```python
from build123d import *

# Parameters (mm, degrees)
BOSS_EXTRUDE1_DEPTH        = 32.1564
SKETCH2_W                  = 57.9628
SKETCH2_H                  = 20.955
CUT_EXTRUDE1_DEPTH         = 80.772
F_31_0_12_DIAMETER_HOLE1_D = 3.048
F_2_0_221_DIAMETER_HOLE1_D = 5.6134
FILLET1_R                  = 2.54


with BuildPart() as part:
    # Sketch1 → Boss-Extrude1 (new body, symmetric)
    with BuildSketch(Plane(origin=(0, 0, 0), x_dir=(0, 0, -1), z_dir=(1, 0, 0))):
        Polygon((0, 0), (24.13, 0), (9.4742, 83.947), (0, 83.947), align=None)
    extrude(amount=BOSS_EXTRUDE1_DEPTH, both=True)

    # Sketch2 → Cut-Extrude1 (cut)
    with BuildSketch(Plane(origin=(0, 83.947, 0), x_dir=(1, 0, 0), z_dir=(0, 1, 0))):
        with Locations((0, 13.6525)):
            Rectangle(SKETCH2_W, SKETCH2_H)
    extrude(amount=-CUT_EXTRUDE1_DEPTH, mode=Mode.SUBTRACT)

    # #31 (0.12) Diameter Hole1 (through all)
    with Locations(Plane.XY):
        with Locations((-21.971, 74.3331), (22.0472, 74.3331), (22.0472, 10.668), (-21.971, 10.668)):
            Hole(F_31_0_12_DIAMETER_HOLE1_D / 2)

    # #2 (0.221) Diameter Hole1 (through all)
    with Locations(Plane(origin=(0, 0, 0), x_dir=(-1, 0, 0), z_dir=(0, -1, 0))):
        with Locations((-16.9164, 12.065), (16.9164, 12.065)):
            Hole(F_2_0_221_DIAMETER_HOLE1_D / 2)

    # Fillet1
    fillet1_edges = [part.edges().sort_by_distance(p)[0] for p in [
        (0, 3.175, -23.575695915),
        (28.9814, 43.561, -16.524947958),
        (-28.9814, 43.561, -16.524947958),
        (-28.9814, 43.561, -3.175),
        (-28.9814, 83.947, -6.3246),
        (0, 83.947, -3.175),
        (28.9814, 83.947, -6.3246),
        (28.9814, 3.175, -13.375347958),
        (0, 3.175, -3.175),
        (-28.9814, 3.175, -13.375347958),
        (28.9814, 43.561, -3.175),
    ]]
    fillet(fillet1_edges, radius=FILLET1_R)


solid = part.part
```
Design review of the part built by this model. Coordinates are the model's own, in mm. A direction names the side the tool comes from. Coordinates: 2 decimals unless noted, no trailing zeros. Order: outer loops, then holes, each group sorted by start corner. A loop starts at its lowest first (then second) coordinate and runs counter-clockwise, first axis right, second up.
1) Mouldability with a two-part tool opening along X and no side actions: class faces 3 (the flat face through (0.2, 83.947, -0.2)), 4 (the flat face through (-32.156, 33, -9)), 5 (the flat face through (-28.981, 36, -11)) as +X half, -X half, draft (parallel to the pull), parting line (faces both ways), or undercut.
2) Take a section at B-B, the plane x = -16. Give the boundary of the cut face in (y, z) (3 decimals).
3) Clearance check with flat-ended pins moving along their axes: pin 1 (12 mm diameter, centred on x = 5.5, z = -19, fed in from +Y) (3 decimals); pin 2 (5 mm diameter, centred on x = 22.05, y = 10.67, fed in from -Z) (3 decimals). State where each tip first meets the part, or that it passes through.
4) For faces 1 (the cylindrical face through (-20.848, 75.363, -1.61)), 2 (the cylindrical face through (29.7, 44.4, -15.6)), list the 3-axis set-ups (+Z, -Z, +X, -X, +Y, -Y) from which the entire face can be reached by the end or side of a thin tool; tool diameter is ignored.
5) Take a section at C-C, the plane z = -13.5. State how many separate pieces and enclosed holes the cut face has, and give its area (3 significant figures).
6) Wall thickness on line 1 along X through (y, z) = (10.5, -11.75); line 2 along Z through (x, y) = (-2.5, 62.5) (3 decimals); line 3 along X through (y, z) = (48, -5): over which ranges is each line inside the solid? List them lowest first.
7) Take a section at A-A, the plane x = -3. Give the boundary of the cut face in (y, z) (3 decimals), and give its area (3 significant figures).
Returned:
1. face 3: draft
1. face 4: -X half
1. face 5: undercut
2. outline: (0, -24.13) - (1.072, -23.943) arc R2.54 ccw to (3.175, -21.441) - (3.175, -14.718) - (0, -14.718) - close; (0, -9.412) - (3.175, -9.412) - (3.175, -5.715) arc R2.54 cw to (5.715, -3.175) - (81.407, -3.175) arc R2.54 ccw to (83.947, -0.635) - (83.947, 0) - (0, 0) - close
3. pin 1: stops at y = 3.175
3. pin 2: stops at z = -3.175
4. face 1: +Z, -Z
4. face 2: -Z, +Y
5. separate pieces: 3
5. enclosed holes: 0
5. area: 527 mm2
6. line 1: x = -32.16 to -28.98, 28.98 to 32.16
6. line 2: z = -3.175 to 0
6. line 3: x = -32.16 to -28.88, 28.88 to 32.16
7. outline: (0, -24.13) - (1.072, -23.943) arc R2.54 ccw to (3.175, -21.441) - (3.175, -5.715) arc R2.54 cw to (5.715, -3.175) - (81.407, -3.175) arc R2.54 ccw to (83.947, -0.635) - (83.947, 0) - (0, 0) - close
7. area: 331 mm2
